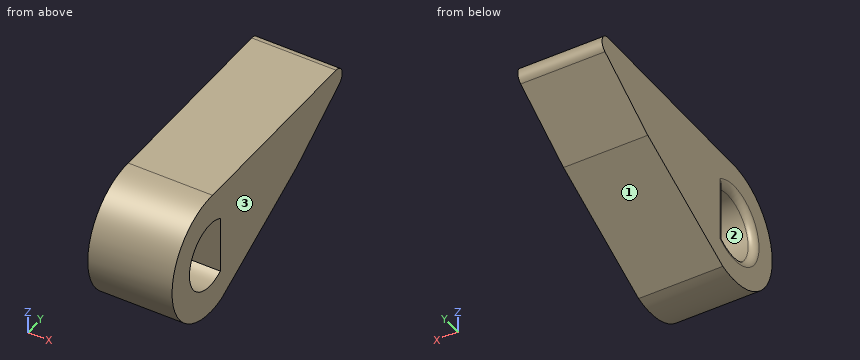
```python
from build123d import *

# Parameters (mm, degrees)
BOSS_EXTRUDE2_DEPTH = 2.5
SKETCH4_R           = 0.99
CUT_EXTRUDE2_DEPTH  = 64.981998238
SKETCH7_W           = 2.01987101
SKETCH7_H           = 0.78494751
BOSS_EXTRUDE5_DEPTH = 2.5
FILLET1_R           = 0.2
BOSS_EXTRUDE6_DEPTH = 2.5
CUT_EXTRUDE5_DEPTH  = 66.492743437
FILLET14_R          = 0.3


with BuildPart() as part:
    # Sketch3 → Boss-Extrude2 (new body)
    with BuildSketch(Plane(origin=(0, 0, 0), x_dir=(0, 0, -1), z_dir=(1, 0, 0))):
        with BuildLine():
            Line((-54.67077374, 30.968825597), (-55.447230875, 28.071048118))
            ThreePointArc((-55.447230875, 28.071048118), (-53.67077374, 25.686416202), (-51.894316605, 28.071048118))
            Line((-51.894316605, 28.071048118), (-52.67077374, 30.968825597))
            ThreePointArc((-52.67077374, 30.968825597), (-53.67077374, 31.692969852), (-54.67077374, 30.968825597))
        make_face()
    extrude(amount=BOSS_EXTRUDE2_DEPTH)

    # Sketch4 → Cut-Extrude2 (cut, through all)
    with BuildSketch(Plane(origin=(2.5, 0, 0), x_dir=(0, 0, -1), z_dir=(1, 0, 0))):
        with Locations((-53.67077374, 27.514195996)):
            Circle(SKETCH4_R)
    extrude(amount=-CUT_EXTRUDE2_DEPTH, mode=Mode.SUBTRACT)

    # Sketch7 → Boss-Extrude5 (add)
    with BuildSketch(Plane(origin=(2.5, 0, 0), x_dir=(0, 0, -1), z_dir=(1, 0, 0))):
        with Locations((-53.657499813, 28.408869671)):
            Rectangle(SKETCH7_W, SKETCH7_H)
    extrude(amount=-BOSS_EXTRUDE5_DEPTH)

    # Fillet1
    fillet1_edges = [part.edges().sort_by_distance(p)[0] for p in [
        (0, 26.524195996, 53.67077374),
        (0, 28.016395916, 53.67077374),
    ]]
    fillet(fillet1_edges, radius=FILLET1_R)

    # Sketch8 → Boss-Extrude6 (add)
    with BuildSketch(Plane(origin=(2.5, 0, 0), x_dir=(0, 0, -1), z_dir=(1, 0, 0))):
        Polygon((-55.522016872, 27.641704373), (-55.522016872, 34.641704373), (-53.67077374, 31.692969852), align=None)
    extrude(amount=-BOSS_EXTRUDE6_DEPTH)

    # Sketch12 → Cut-Extrude5 (cut, through all)
    with BuildSketch(Plane(origin=(2.5, 0, 0), x_dir=(0, 0, -1), z_dir=(1, 0, 0))):
        Polygon((-53.67077374, 31.692969852), (-51.894316605, 28.071048118), (-51.781619292, 31.692969852), align=None)
    extrude(amount=-CUT_EXTRUDE5_DEPTH, mode=Mode.SUBTRACT)

    # Fillet14
    fillet14_edges = [part.edges().sort_by_distance(p)[0] for p in [
        (1.25, 34.641704373, 55.522016872),
    ]]
    fillet(fillet14_edges, radius=FILLET14_R)


solid = part.part
```
Input: part model. Units: mm. Frame: model coordinates. Face numbers are marked on the shaded views. Round coordinates to 2 decimals unless told otherwise and drop trailing zeros. Loops run counter-clockwise (first coordinate to the right, second up) from the corner with the lowest first, then second, coordinate; pieces in that order, holes last.
1) Pull-direction query (Y, two-part tool) for the marked faces 1, 2 and 3; classes: released by +Y, released by -Y, zero draft, split by the parting line, or undercut.
Ans:
face 1: released by +Y
face 2: undercut
face 3: zero draft
2) Material intervals for line 1 (Y direction, x = 2, z = 53.7); line 2 (Y direction, x = 2.2, z = 53); line 3 (Z direction, x = 0.95, y = 26.75), sorted ascending.
Ans:
line 1: y = 25.69 to 26.52, 28.02 to 31.74
line 2: y = 25.81 to 26.79, 28.02 to 30.33
line 3: z = 51.99 to 53.04, 54.3 to 55.35
3) Section query A-A on x = 1.1. Return the cut outline in (y, z).
Ans:
outline: (27.64, 55.52) arc R1.85 ccw (long way) to (28.07, 51.89) - (31.69, 53.67) - (33.76, 54.97) arc R0.3 ccw to (33.6, 55.52) - close; hole (28.02, 52.82) - (28.02, 54.52) arc R0.99 ccw (long way) to start
4) Pin query (flat end, axial travel): pin 1 (1.6 mm diameter, centred on y = 27.51, z = 53.67, fed in from -X); pin 2 (0.8 mm diameter, centred on x = 1, y = 31, fed in from +Z). Return the tip coordinate at first contact, or that it passes through.
Ans:
pin 1: stops at x = 0
pin 2: stops at z = 55.52
5) Section query B-B on z = 52.4. Return the cut outline in (x, y).
Ans:
outline: (0, 26.19) - (2.5, 26.19) - (2.5, 29.1) - (0, 29.1) - close
6) Section query C-C on y = 33. Return the cut outline in (x, z), plus the area to 3 significant figures.
Ans:
outline: (0, 54.49) - (2.5, 54.49) - (2.5, 55.52) - (0, 55.52) - close
area: 2.58 mm2
